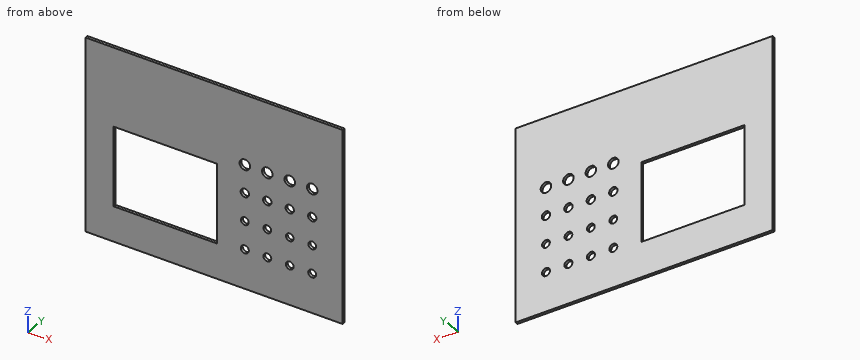
```python
from build123d import *

# Parameters (mm, degrees)
SKETCH1_W           = 581.66
SKETCH1_H           = 436.88
BOSS_EXTRUDE1_DEPTH = 6.35
SKETCH3_W           = 233.426
SKETCH3_H           = 179.578
CUT_EXTRUDE2_DEPTH  = 728.483891574
SKETCH4_R           = 9.017
CUT_EXTRUDE3_DEPTH  = 728.483891574
SKETCH5_R           = 8.763
CUT_EXTRUDE4_DEPTH  = 728.483891574
SKETCH6_R           = 9.525
CUT_EXTRUDE5_DEPTH  = 728.483891574
SKETCH7_R           = 11.938
CUT_EXTRUDE6_DEPTH  = 728.483891574


with BuildPart() as part:
    # Sketch1 → Boss-Extrude1 (new body)
    with BuildSketch(Plane(origin=(0, 0, 0), x_dir=(1, 0, 0), z_dir=(0, 1, 0))):
        with Locations((290.83, 218.44)):
            Rectangle(SKETCH1_W, SKETCH1_H)
    extrude(amount=BOSS_EXTRUDE1_DEPTH)

    # Sketch3 → Cut-Extrude2 (cut, through all)
    with BuildSketch(Plane(origin=(0, 6.35, 0), x_dir=(1, 0, 0), z_dir=(0, 1, 0))):
        with Locations((180.213, 267.589)):
            Rectangle(SKETCH3_W, SKETCH3_H)
    extrude(amount=-CUT_EXTRUDE2_DEPTH, mode=Mode.SUBTRACT)

    # Sketch4 → Cut-Extrude3 (cut, through all)
    with BuildSketch(Plane(origin=(0, 6.35, 0), x_dir=(1, 0, 0), z_dir=(0, 1, 0))):
        with Locations(Location((360.426, 347.98, 0), (0, 0, 270))):
            Circle(SKETCH4_R)
        with Locations(Location((411.226, 347.98, 0), (0, 0, 270))):
            Circle(SKETCH4_R)
        with Locations(Location((462.026, 347.98, 0), (0, 0, 270))):
            Circle(SKETCH4_R)
        with Locations(Location((512.826, 347.98, 0), (0, 0, 270))):
            Circle(SKETCH4_R)
    extrude(amount=-CUT_EXTRUDE3_DEPTH, mode=Mode.SUBTRACT)

    # Sketch5 → Cut-Extrude4 (cut, through all)
    with BuildSketch(Plane(origin=(0, 6.35, 0), x_dir=(1, 0, 0), z_dir=(0, 1, 0))):
        with Locations(Location((360.426, 284.48, 0), (0, 0, 270))):
            Circle(SKETCH5_R)
        with Locations(Location((411.226, 284.48, 0), (0, 0, 270))):
            Circle(SKETCH5_R)
        with Locations(Location((462.026, 284.48, 0), (0, 0, 270))):
            Circle(SKETCH5_R)
        with Locations(Location((512.826, 284.48, 0), (0, 0, 270))):
            Circle(SKETCH5_R)
    extrude(amount=-CUT_EXTRUDE4_DEPTH, mode=Mode.SUBTRACT)

    # Sketch6 → Cut-Extrude5 (cut, through all)
    with BuildSketch(Plane(origin=(0, 6.35, 0), x_dir=(1, 0, 0), z_dir=(0, 1, 0))):
        with Locations(Location((360.426, 220.98, 0), (0, 0, 270))):
            Circle(SKETCH6_R)
        with Locations(Location((411.226, 220.98, 0), (0, 0, 270))):
            Circle(SKETCH6_R)
        with Locations(Location((462.026, 220.98, 0), (0, 0, 270))):
            Circle(SKETCH6_R)
        with Locations(Location((512.826, 220.98, 0), (0, 0, 270))):
            Circle(SKETCH6_R)
    extrude(amount=-CUT_EXTRUDE5_DEPTH, mode=Mode.SUBTRACT)

    # Sketch7 → Cut-Extrude6 (cut, through all)
    with BuildSketch(Plane(origin=(0, 6.35, 0), x_dir=(1, 0, 0), z_dir=(0, 1, 0))):
        with Locations(Location((360.426, 157.48, 0), (0, 0, 270))):
            Circle(SKETCH7_R)
        with Locations(Location((411.226, 157.48, 0), (0, 0, 270))):
            Circle(SKETCH7_R)
        with Locations(Location((462.026, 157.48, 0), (0, 0, 270))):
            Circle(SKETCH7_R)
        with Locations(Location((512.826, 157.48, 0), (0, 0, 270))):
            Circle(SKETCH7_R)
    extrude(amount=-CUT_EXTRUDE6_DEPTH, mode=Mode.SUBTRACT)


solid = part.part
```
Input: part model. Units: mm. Frame: model coordinates. Give positions to 0.01 mm unless a question says otherwise; leave off trailing zeros. Write each loop counter-clockwise with the first axis right and the second up, starting at its lowest first coordinate (ties: lowest second). Pieces come first, ordered by that corner, then holes. Notation, with made-up numbers: (30.5, 10) - (74.5, 10) arc R23 ccw to (74.5, 42) - close; hole circle Ø5 at (24, 37.25). An arc over 180 degrees is marked (long way). Write item = value, one per line. Start each with the question number.
1) Cut plane D-D (y = 3). Give the number of separate pieces and of enclosed holes in the cut face, and give its area (3 significant figures).
2) Cut plane C-C (x = 91). Return loops of the section in (y, z), and give its area (3 significant figures).
3) Cut plane B-B (z = -157.48). Return loops of the section in (x, y), and give its area (3 significant figures).
4) Pin query (flat end, axial travel): pin 1 (14.5 mm diameter, centred on x = 360.426, z = -347.98, fed in from -Y). Return the tip coordinate at first contact, or that it passes through.
5) Material intervals for L1, parallel to X at y = 4.25, z = -220.98; L2, parallel to X at y = 2.25, z = -157.48; L3, parallel to Z at x = 356, y = 6.25, sorted ascending. Write a range as [from, to].
6) Cut plane A-A (z = -347.98). Return loops of the section in (x, y).
Answers follow:
q1.separate_pieces = 1
q1.enclosed_holes = 17
q1.area = 207,000 mm^2
q2.outline = (0, -436.88) - (6.35, -436.88) - (6.35, -357.38) - (0, -357.38) - close; (0, -177.8) - (6.35, -177.8) - (6.35, 0) - (0, 0) - close
q2.area = 1,630 mm^2
q3.outline = (0, 0) - (348.49, 0) - (348.49, 6.35) - (0, 6.35) - close; (372.36, 0) - (399.29, 0) - (399.29, 6.35) - (372.36, 6.35) - close; (423.16, 0) - (450.09, 0) - (450.09, 6.35) - (423.16, 6.35) - close; (473.96, 0) - (500.89, 0) - (500.89, 6.35) - (473.96, 6.35) - close; (524.76, 0) - (581.66, 0) - (581.66, 6.35) - (524.76, 6.35) - close
q3.area = 3,090 mm^2
q4.pin_1 = through
q5.L1 = [0, 63.5], [296.93, 350.9], [369.95, 401.7], [420.75, 452.5], [471.55, 503.3], [522.35, 581.66]
q5.L2 = [0, 348.49], [372.36, 399.29], [423.16, 450.09], [473.96, 500.89], [524.76, 581.66]
q5.L3 = [-436.88, -355.84], [-340.12, -292.04], [-276.92, -229.41], [-212.55, -168.57], [-146.39, 0]
q6.outline = (0, 0) - (63.5, 0) - (63.5, 6.35) - (0, 6.35) - close; (296.93, 0) - (351.41, 0) - (351.41, 6.35) - (296.93, 6.35) - close; (369.44, 0) - (402.21, 0) - (402.21, 6.35) - (369.44, 6.35) - close; (420.24, 0) - (453.01, 0) - (453.01, 6.35) - (420.24, 6.35) - close; (471.04, 0) - (503.81, 0) - (503.81, 6.35) - (471.04, 6.35) - close; (521.84, 0) - (581.66, 0) - (581.66, 6.35) - (521.84, 6.35) - close
